from build123d import *

# Parameters (mm, degrees)
SKETCH1_W           = 409.5
SKETCH1_H           = 335
BOSS_EXTRUDE1_DEPTH = 3
SKETCH1_3_W         = 110
SKETCH1_3_H         = 52
BOSS_EXTRUDE2_DEPTH = 28
SKETCH1_6_W         = 53.5
SKETCH1_6_H         = 100
SKETCH1_6_W_2       = 30
SKETCH1_6_H_2       = 87
SKETCH1_6_W_3       = 56
BOSS_EXTRUDE3_DEPTH = 48
SKETCH1_7_W         = 48
SKETCH1_7_H         = 85
BOSS_EXTRUDE4_DEPTH = 38
BOSS_EXTRUDE5_DEPTH = 55
SKETCH1_9_W         = 6
SKETCH1_9_H         = 44
BOSS_EXTRUDE6_DEPTH = 38
SKETCH1_10_W        = 15
SKETCH1_10_H        = 15
BOSS_EXTRUDE7_DEPTH = 6


with BuildPart() as part:
    # Sketch1 → Boss-Extrude1 (new body)
    with BuildSketch(Plane(origin=(0, 0, 0), x_dir=(0, 0, -1), z_dir=(1, 0, 0))):
        with Locations((-15.25, -17.5)):
            Rectangle(SKETCH1_W, SKETCH1_H)
    extrude(amount=BOSS_EXTRUDE1_DEPTH)

    # Sketch1_3 → Boss-Extrude2 (add)
    with BuildSketch(Plane(origin=(0, 0, 0), x_dir=(0, 0, -1), z_dir=(1, 0, 0))):
        with Locations((-115, 74)):
            Rectangle(SKETCH1_3_W, SKETCH1_3_H)
        with Locations((-115, -8)):
            Rectangle(SKETCH1_3_W, SKETCH1_3_H)
        with Locations((-115, -90)):
            Rectangle(SKETCH1_3_W, SKETCH1_3_H)
    extrude(amount=BOSS_EXTRUDE2_DEPTH)

    # Sketch1_6 → Boss-Extrude3 (add)
    with BuildSketch(Plane(origin=(0, 0, 0), x_dir=(0, 0, -1), z_dir=(1, 0, 0))):
        with Locations((26.75, 50)):
            Rectangle(SKETCH1_6_W, SKETCH1_6_H)
        with Locations((68.5, 56.5)):
            Rectangle(SKETCH1_6_W_2, SKETCH1_6_H_2)
        with Locations((111.5, 56.5)):
            Rectangle(SKETCH1_6_W_3, SKETCH1_6_H_2)
    extrude(amount=BOSS_EXTRUDE3_DEPTH)

    # Sketch1_7 → Boss-Extrude4 (add)
    with BuildSketch(Plane(origin=(0, 0, 0), x_dir=(0, 0, -1), z_dir=(1, 0, 0))):
        with Locations((30, -92.5)):
            Rectangle(SKETCH1_7_W, SKETCH1_7_H)
    extrude(amount=BOSS_EXTRUDE4_DEPTH)

    # Sketch1_8 → Boss-Extrude5 (add)
    with BuildSketch(Plane(origin=(0, 0, 0), x_dir=(0, 0, -1), z_dir=(1, 0, 0))):
        Polygon((54, -47.5), (54, -50), (54, -135), (54, -137.5), (100.5, -137.5), (100.5, -114.5), (100.5, -70.5), (100.5, -47.5), align=None)
    extrude(amount=BOSS_EXTRUDE5_DEPTH)

    # Sketch1_9 → Boss-Extrude6 (add)
    with BuildSketch(Plane(origin=(0, 0, 0), x_dir=(0, 0, -1), z_dir=(1, 0, 0))):
        with Locations((103.5, -92.5)):
            Rectangle(SKETCH1_9_W, SKETCH1_9_H)
        with Locations((3, -92.5)):
            Rectangle(SKETCH1_9_W, SKETCH1_9_H)
    extrude(amount=BOSS_EXTRUDE6_DEPTH)

    # Sketch1_10 → Boss-Extrude7 (add)
    with BuildSketch(Plane(origin=(0, 0, 0), x_dir=(0, 0, -1), z_dir=(1, 0, 0))):
        with Locations((-197.5, 92.5)):
            Rectangle(SKETCH1_10_W, SKETCH1_10_H)
        with Locations((-197.5, -127.5)):
            Rectangle(SKETCH1_10_W, SKETCH1_10_H)
        with Locations((-197.5, -52.5)):
            Rectangle(SKETCH1_10_W, SKETCH1_10_H)
        with Locations((-197.5, 17.5)):
            Rectangle(SKETCH1_10_W, SKETCH1_10_H)
        with Locations((-162.5, -162.5)):
            Rectangle(SKETCH1_10_W, SKETCH1_10_H)
        with Locations((-87.5, -162.5)):
            Rectangle(SKETCH1_10_W, SKETCH1_10_H)
        with Locations((-12.5, -162.5)):
            Rectangle(SKETCH1_10_W, SKETCH1_10_H)
        with Locations((132, -162.5)):
            Rectangle(SKETCH1_10_W, SKETCH1_10_H)
        with Locations((57, -162.5)):
            Rectangle(SKETCH1_10_W, SKETCH1_10_H)
        with Locations((167, 92.5)):
            Rectangle(SKETCH1_10_W, SKETCH1_10_H)
        with Locations((167, 17.5)):
            Rectangle(SKETCH1_10_W, SKETCH1_10_H)
        with Locations((167, -52.5)):
            Rectangle(SKETCH1_10_W, SKETCH1_10_H)
        with Locations((167, -127.5)):
            Rectangle(SKETCH1_10_W, SKETCH1_10_H)
        with Locations((-162.5, 127.5)):
            Rectangle(SKETCH1_10_W, SKETCH1_10_H)
        with Locations((-87.5, 127.5)):
            Rectangle(SKETCH1_10_W, SKETCH1_10_H)
        with Locations((57, 127.5)):
            Rectangle(SKETCH1_10_W, SKETCH1_10_H)
        with Locations((132, 127.5)):
            Rectangle(SKETCH1_10_W, SKETCH1_10_H)
        with Locations((-12.5, 127.5)):
            Rectangle(SKETCH1_10_W, SKETCH1_10_H)
    extrude(amount=BOSS_EXTRUDE7_DEPTH)


solid = part.part
Check sheet for the modelled part. Datum: model origin and axes. Units: mm. A direction names the side the tool comes from. Round coordinates to 2 decimals unless told otherwise and drop trailing zeros. Order: outer loops, then holes, each group sorted by start corner. A loop starts at its lowest first (then second) coordinate and runs counter-clockwise, first axis right, second up.
Q1. Cross-section at B-B, the plane z = -16.5. Enter the section's corners in (x, y), plus the area to 3 significant figures.
Filled sheet:
outline: (0, -185) - (3, -185) - (3, -135) - (38, -135) - (38, -50) - (3, -50) - (3, 0) - (48, 0) - (48, 100) - (3, 100) - (3, 150) - (0, 150) - close
area: 8,480 mm2
Q2. Draft check along Z on faces 6 (the face through (15, -90, 60)), 7 (the face through (20, -93, -106.5)), 8 (the face through (6, 93, 198)). Enter one of: pulls with the +Z half, pulls with the -Z half, needs draft (parallel to the pull), parting line crosses it, or undercut.
Filled sheet:
face 6: undercut
face 7: pulls with the -Z half
face 8: needs draft
Q3. Cross-section at C-C, the plane y = 61.5. Enter the section's corners in (x, z).
Filled sheet:
outline: (0, -189.5) - (3, -189.5) - (3, -139.5) - (48, -139.5) - (48, 0) - (3, 0) - (3, 60) - (28, 60) - (28, 170) - (3, 170) - (3, 220) - (0, 220) - close
Q4. Set-up check for faces 1 (the face through (6, -162, -57)), 2 (the face through (25, 0, -26)), 3 (the face through (6, 128, -132)), 4 (the face through (6, 93, -167)), 5 (the face through (6, -52, 198)): record each of +Z, -Z, +X, -X, +Y, -Y from which the full face is reachable in a straight line by a thin tool's end or side.
Filled sheet:
face 1: +Z, -Z, +X, -Y
face 2: -Z, +X
face 3: +Z, -Z, +X, +Y
face 4: -Z, +X, +Y, -Y
face 5: +Z, +X, +Y, -Y
Q5. Cross-section at A-A, the plane x = 42.5. Enter the section's corners in (y, z).
Filled sheet:
outline: (-137.5, -100.5) - (-47.5, -100.5) - (-47.5, -54) - (-137.5, -54) - close; (0, -53.5) - (13, -53.5) - (13, -139.5) - (100, -139.5) - (100, 0) - (0, 0) - close
Q6. Cross-section at D-D, the plane x = 20.5. Give the number of separate pieces and of enclosed holes in the cut face, plus the area to 3 significant figures.
Filled sheet:
separate pieces: 5
enclosed holes: 0
area: 38,800 mm2
Q7. Depth check by flat-ended pin: P1, Ø16.5, axis at x = 14.5, y = -59.5, coming from the +Z side; P2, Ø3.5, axis at x = 5, y = -54.5, coming from the +Z side; P3, Ø6, axis at x = 12.5, z = -18, coming from the -Y side; P4, Ø1.5, axis at y = 86.5, z = 143, coming from the -X side. Enter the tip coordinate at first touch or a pass-through.
Filled sheet:
P1: stops at z = 170
P2: stops at z = 205
P3: stops at y = -135
P4: stops at x = 0
Q8. Scan lines: L1, parallel to Z at x = 22.5, y = -80.5; L2, parallel to Z at x = 20, y = 6; L3, parallel to Y at x = 12, z = -64.5. Record each from-to range of solid material in increasing order.
Filled sheet:
L1: z = -106.5 to 0, 60 to 170
L2: z = -53.5 to 0, 60 to 170
L3: y = -137.5 to -47.5, 13 to 100
